Autodesk Inventor part; units mm, degrees
ref_plane "YZ Plane" through (0, 0, 0) normal (1, 0, 0) x (0, 1, 0)
ref_plane "XZ Plane" through (0, 0, 0) normal (0, 1, 0) x (-1, 0, 0)
ref_plane "XY Plane" through (0, 0, 0) normal (0, 0, 1) x (1, 0, 0)
sketch "Sketch1" plane through (0, 0, 0) normal (0, 1, 0) x (-1, 0, 0)
  point P0 (0, 0)
sketch "Sketch2" plane through (0, 0, 0) normal (0, 1, 0) x (-1, 0, 0)
  line L0 (-140.5, 177) -> (140.5, 177)
  line L1 (140.5, 177) -> (140.5, -177)
  line L2 (140.5, -177) -> (-140.5, -177)
  line L3 (-140.5, -177) -> (-140.5, 177)
  line L4 (-140.5, 177) -> (140.5, -177) construction
  line L5 (140.5, 177) -> (-140.5, -177) construction
  point P0 (0, 0)
  dimension "d0" = 354
  dimension "d1" = 281
extrude "Extrusion1" add sketch "Sketch2" along normal blind 11.4
sketch "Sketch3" plane through (0, 0, 0) normal (0, -1, 0) x (1, 0, 0)
  line L0 (-124, -160.5) -> (125.8, -160.5)
  line L1 (125.8, -160.5) -> (125.8, 160.5)
  line L2 (125.8, 160.5) -> (-124, 160.5)
  line L3 (-124, 160.5) -> (-124, -160.5)
  line L4 (-123, -158.8) -> (123, 158.8) construction
  line L5 (123, -158.8) -> (-123, 158.8) construction
  circle A0 centre (-115.5, -152) radius 2
  circle A1 centre (117.3, -152) radius 2
  circle A2 centre (117.3, 152) radius 2
  circle A3 centre (-115.5, 152) radius 2
  line L6 (-140.5, -177) -> (-140.5, 177)
  line L7 (-140.5, 177) -> (140.5, 177)
  line L8 (140.5, -177) -> (-140.5, -177)
  line L9 (140.5, 177) -> (140.5, -177)
  circle A4 centre (-115.5, 0) radius 2
  circle A5 centre (117.3, 0) radius 2
  circle A6 centre (0, 152) radius 2
  circle A7 centre (0, -152) radius 2
  point P0 (0, 0)
  dimension "d189" = 4
  dimension "d190" = 8.5
  dimension "d191" = 8.5
  dimension "d192" = 8.5
  dimension "d193" = 8.5
  dimension "d194" = 8.5
  dimension "d195" = 8.5
  dimension "d196" = 8.5
  dimension "d197" = 8.5
  dimension "d207" = 16.5
  dimension "d208" = 16.5
  dimension "d209" = 16.5
  dimension "d210" = 14.7
  dimension "d211" = 8.5
  dimension "d212" = 354
  dimension "d213" = 177
  dimension "d214" = 8.5
  dimension "d215" = 177
  dimension "d216" = 8.5
  dimension "d217" = 281
  dimension "d218" = 140.5
  dimension "d220" = 140.5
  dimension "d221" = 8.5
extrude "Extrusion2" add sketch "Sketch3" along normal blind 12 contours L3 L2 L1 L0
sketch "Sketch7" plane through (0, -12, 0) normal (0, -1, 0) x (1, 0, 0)
  line L0 (-52.5, 141) -> (105.5, 141)
  line L1 (105.5, 141) -> (105.5, -141)
  line L2 (105.5, -141) -> (-52.5, -141)
  line L3 (-52.5, -141) -> (-52.5, 141)
  line L4 (-52.5, 141) -> (105.5, -141) construction
  line L5 (105.5, 141) -> (-52.5, -141) construction
  line L6 (125.8, -160.5) -> (125.8, 160.5)
  line L7 (-124, -160.5) -> (125.8, -160.5)
  line L8 (-140.5, 177) -> (140.5, 177)
  line L9 (140.5, -177) -> (-140.5, -177)
  line L10 (140.5, 177) -> (140.5, -177)
  point P0 (0, 0)
  dimension "d62" = 158
  dimension "d204" = 36
  dimension "d205" = 36
  dimension "d206" = 35
extrude "Extrusion3" add sketch "Sketch7" along normal blind 31.2
sketch "Sketch8" plane through (0, -43.2, 0) normal (0, -1, 0) x (1, 0, 0)
  line L0 (99.2, 131) -> (81.2, 131)
  line L1 (81.2, 131) -> (81.2, 15)
  line L2 (81.2, 15) -> (99.2, 15)
  line L3 (99.2, 15) -> (99.2, 131)
  line L4 (99.2, 131) -> (81.2, 15) construction
  line L5 (81.2, 131) -> (99.2, 15) construction
  line L6 (105.5, -141) -> (105.5, 141)
  line L7 (105.5, 141) -> (-52.5, 141)
  point P0 (0, 0)
  point P1 (90.2, 73)
  dimension "d67" = 116
  dimension "d68" = 18
  dimension "d69" = 6.3
  dimension "d70" = 10
extrude "Extrusion4" add sketch "Sketch8" along normal blind 1
sketch "Sketch9" plane through (0, -43.2, 0) normal (0, -1, 0) x (1, 0, 0)
  line L0 (100, -71.4) -> (42.15, -71.4)
  line L1 (42.15, -71.4) -> (42.15, -129.25)
  line L2 (42.15, -129.25) -> (100, -129.25)
  line L3 (100, -129.25) -> (100, -71.4)
  line L4 (100, -71.4) -> (42.15, -129.25) construction
  line L5 (42.15, -71.4) -> (100, -129.25) construction
  line L6 (105.5, -141) -> (105.5, 141)
  line L7 (-52.5, -141) -> (105.5, -141)
  point P0 (0, 0)
  point P1 (71.075, -100.325)
  dimension "d73" = 5.5
  dimension "d74" = 57.85
  dimension "d75" = 11.75
  dimension "d76" = 57.85
extrude "Extrusion5" add sketch "Sketch9" along normal blind 1
sketch "Sketch10" plane through (0, -43.2, 0) normal (0, -1, 0) x (1, 0, 0)
  line L0 (105.5, 141) -> (-52.5, 141)
  line L1 (-52.5, 141) -> (-52.5, -141)
  line L2 (-52.5, -141) -> (105.5, -141)
  point P0 (0, 0)
  point P1 (-45.5, 120.2)
  point P2 (-45.5, -119.9)
  dimension "d86" = 20.8
  dimension "d87" = 7
  dimension "d90" = 240.1
  dimension "d95" = 21.1
hole "Hole4" at (-45.5, -43.2, 120.2) at (-45.5, -43.2, -119.9) direction (0, 1, 0) diameter 7 depth 8 tip angle 118
sketch "Sketch11" plane through (0, -43.2, 0) normal (0, -1, 0) x (1, 0, 0)
  line L0 (105.5, 141) -> (-52.5, 141)
  line L1 (-52.5, 141) -> (-52.5, -141)
  line L2 (125.8, 160.5) -> (-124, 160.5)
  point P0 (0, 0)
  point P1 (-45.5, 0)
  dimension "d103" = 141
  dimension "d104" = 7
  dimension "d185" = 160.5
hole "Hole5" at (-45.5, -43.2, 0) direction (0, 1, 0) diameter 7 depth 8 tip angle 118
sketch "Sketch12" plane through (0, -43.2, 0) normal (0, -1, 0) x (1, 0, 0)
  line L0 (105.5, 141) -> (-52.5, 141)
  line L1 (-52.5, 141) -> (-52.5, -141)
  point P0 (0, 0)
  point P1 (-18.7, 37.65)
  point P2 (-18.7, -36.85)
  point P3 (55.8, 37.65)
  point P4 (55.8, -36.85)
  dimension "d112" = 103.35
  dimension "d113" = 33.8
  dimension "d116" = 74.5
  dimension "d119" = 74.5
hole "Hole6" at (-18.7, -43.2, 37.65) at (55.8, -43.2, 37.65) at (55.8, -43.2, -36.85) at (-18.7, -43.2, -36.85) direction (0, 1, 0) diameter 7 depth 8 tip angle 118
sketch "Sketch13" plane through (-52.5, -12, -141) normal (-1, 0, 0) x (0, 0, 1)
  line L0 (223, -24.2) -> (195.5, -24.2)
  line L1 (195.5, -24.2) -> (195.5, -2.2)
  line L2 (195.5, -2.2) -> (223, -2.2)
  line L3 (223, -2.2) -> (223, -24.2)
  line L4 (223, -24.2) -> (195.5, -2.2) construction
  line L5 (195.5, -24.2) -> (223, -2.2) construction
  line L6 (282, 0) -> (282, -31.2)
  line L7 (282, -31.2) -> (0, -31.2)
  point P0 (141, 12)
  point P1 (209.25, -13.2)
  dimension "d122" = 59
  dimension "d123" = 27.5
  dimension "d124" = 22
  dimension "d133" = 7
extrude "Extrusion6" cut sketch "Sketch13" against normal blind 10
sketch "Sketch14" plane through (-52.5, -12, -141) normal (-1, 0, 0) x (0, 0, 1)
  line L0 (142, -11.8) -> (125, -11.8)
  line L1 (125, -11.8) -> (125, -5.6)
  line L2 (125, -5.6) -> (142, -5.6)
  line L3 (142, -5.6) -> (142, -11.8)
  line L4 (142, -11.8) -> (125, -5.6) construction
  line L5 (125, -11.8) -> (142, -5.6) construction
  line L6 (195.5, -24.2) -> (195.5, -2.2)
  line L7 (282, -31.2) -> (0, -31.2)
  line L8 (223, -24.2) -> (195.5, -24.2)
  line L9 (301.5, 0) -> (-19.5, 0)
  line L10 (195.5, -2.2) -> (223, -2.2)
  line L11 (282, 0) -> (282, -31.2)
  point P0 (141, 12)
  point P1 (133.5, -8.7)
  dimension "d128" = 6.2
  dimension "d129" = 17
  dimension "d130" = 19.4
  dimension "d222" = 140
extrude "Extrusion7" cut sketch "Sketch14" against normal blind 1.5
sketch "Sketch15" plane through (-52.5, -12, -141) normal (-1, 0, 0) x (0, 0, 1)
  line L0 (118, -11.8) -> (103, -11.8)
  line L1 (103, -11.8) -> (103, -5.6)
  line L2 (103, -5.6) -> (118, -5.6)
  line L3 (118, -5.6) -> (118, -11.8)
  line L4 (118, -11.8) -> (103, -5.6) construction
  line L5 (103, -11.8) -> (118, -5.6) construction
  line L6 (125, -11.8) -> (125, -5.6)
  line L7 (282, -31.2) -> (0, -31.2)
  point P0 (141, 12)
  point P1 (110.5, -8.7)
  dimension "d136" = 7
  dimension "d137" = 6.2
  dimension "d138" = 15
  dimension "d141" = 19.4
extrude "Extrusion8" cut sketch "Sketch15" against normal blind 1.5
sketch "Sketch16" plane through (-52.5, -12, -141) normal (-1, 0, 0) x (0, 0, 1)
  circle A0 centre (92.5, -12.2) radius 2.5
  line L0 (103, -11.8) -> (103, -5.6)
  line L1 (282, -31.2) -> (0, -31.2)
  circle A1 centre (68, -12.2) radius 2.5
  line L2 (88.375, -16.2) -> (72.125, -16.2)
  line L3 (72.125, -16.2) -> (72.125, -8.2)
  line L4 (72.125, -8.2) -> (88.375, -8.2)
  line L5 (88.375, -8.2) -> (88.375, -16.2)
  line L6 (88.375, -16.2) -> (72.125, -8.2) construction
  line L7 (72.125, -16.2) -> (88.375, -8.2) construction
  point P0 (141, 12)
  point P1 (80.25, -12.2)
  dimension "d142" = 10.5
  dimension "d144" = 5
  dimension "d147" = 24.5
  dimension "d223" = 19
  dimension "d224" = 12.25
  dimension "d225" = 19
  dimension "d226" = 16.25
  dimension "d227" = 8
extrude "Extrusion9" add sketch "Sketch16" along normal blind 5
sketch "Sketch20" plane through (0, -12, 0) normal (0, -1, 0) x (1, 0, 0)
  circle A0 centre (-59, 120) radius 2
  circle A1 centre (-59, 0) radius 2
  circle A2 centre (-59, -120) radius 2
  line L0 (-52.5, -141) -> (-52.5, 141)
  circle A3 centre (-115.5, 152) radius 2
  point P0 (0, 0)
  dimension "d228" = 21
  dimension "d229" = 6.5
  dimension "d230" = 6.5
  dimension "d231" = 6.5
  dimension "d232" = 21
  dimension "d233" = 240
  dimension "d234" = 120
extrude "Extrusion11" cut sketch "Sketch20" against normal blind 10 contours A0 | A1 | A2
equation "\"d191\" = d190"
equation "\"d192\" = d190"
equation "\"d193\" = d190"
equation "\"d194\" = d190"
equation "\"d195\" = d190"
equation "\"d196\" = d190"
equation "\"d197\" = d190"
equation "\"d209\" = d208"
equation "\"d211\" = d190"
equation "\"d213\" = 0.5 * d212"
equation "\"d214\" = d190"
equation "\"d215\" = d213"
equation "\"d216\" = d190"
equation "\"d218\" = 0.5 * d217"
equation "\"d220\" = d218"
equation "\"d221\" = d190"
equation "\"d205\" = d204"
equation "\"d230\" = d229"
equation "\"d231\" = d229"
equation "\"d232\" = d228"
equation "\"d234\" = 0.5 * d233"
properties part number "LCDScreen"
The listing builds one solid part. Answer for the finished solid, in the listing's coordinates (mm). A direction names the side the tool comes from. Give positions to 0.01 mm unless a question says otherwise; leave off trailing zeros. Loops run counter-clockwise (first coordinate to the right, second up) from the corner with the lowest first, then second, coordinate; pieces in that order, holes last. Notation, with made-up numbers: M 89,-0.5 L 104,-0.5 A32 ccw 104,25.5 Z; hole C -18,-19.5 d10. An arc over 180 degrees is marked long. One line per item, written item: value.
Q1. Find the intervals of material crossed by line 1 (X direction, y = -8.5, z = 152); line 2 (Z direction, x = -59, y = -5.75); line 3 (Z direction, x = 117.3, y = -3.5), in increasing order. Write a range as from..to.
Working result:
line 1: x = -124..-117.5, -113.5..-2, 2..115.3, 119.3..125.8
line 2: z = -160.5..-122, -118..-2, 2..118, 122..160.5
line 3: z = -160.5..-154, -150..-2, 2..150, 154..160.5
Q2. A cutting plane is placed at D-D on z = 25. Determine the outline of the cut face in (x, y).
Working result:
outline: M -140.5,0 L -124,0 L -124,-12 L -52.5,-12 L -52.5,-43.2 L 81.2,-43.2 L 81.2,-44.2 L 99.2,-44.2 L 99.2,-43.2 L 105.5,-43.2 L 105.5,-12 L 125.8,-12 L 125.8,0 L 140.5,0 L 140.5,11.4 L -140.5,11.4 Z
Q3. Determine the mould class of faces 1 (the face through (-45.73, -33.46, -120.46)), 2 (the face through (56.4, -33.46, 37.73)), 3 (the face through (2, 6, 177)), 4 (the face through (-124.2, 0, -12.3)) for opening direction Z: +Z half, -Z half, draft (parallel to the pull), parting line (faces both ways), or undercut.
Working result:
face 1: undercut
face 2: undercut
face 3: +Z half
face 4: draft
Q4. A cutting plane is placed at C-C on z = 135. Determine the outline of the cut face in (x, y), then the cut area to 3 significant figures.
Working result:
outline: M -140.5,0 L -124,0 L -124,-12 L -52.5,-12 L -52.5,-43.2 L 105.5,-43.2 L 105.5,-12 L 125.8,-12 L 125.8,0 L 140.5,0 L 140.5,11.4 L -140.5,11.4 Z
area: 11,100 mm^2
Q5. For faces 5 (the face through (90, -44.2, 74)), 6 (the face through (25, -27, 141)), 7 (the face through (-140.5, 6, 2)), 8 (the face through (-15.595, -39.144, -38.465)), 9 (the face through (-48, -36.2, 68)), determine the directions among +Z, -Z, +X, -X, +Y, -Y from which every point of the face is accessible in a straight line to the end or side of a thin tool.
Working result:
face 5: +Z, -Z, +X, -X, -Y
face 6: +Z, +X, -X, -Y
face 7: +Z, -Z, -X, +Y, -Y
face 8: -Y
face 9: -X
Q6. Flat-ended cylindrical pins translate along their axes: P1, Ø4, axis at y = -23.5, z = -49, coming from the -X side; P2, Ø1.1, axis at x = 86.5, y = -44, coming from the +Z side; P3, Ø0.5, axis at y = -43.5, z = 67.5, coming from the +X side. Find the tip coordinate at first contact, or state that the pin passes through.
Working result:
P1: stops at x = -57.5
P2: stops at z = 131
P3: stops at x = 99.2
Q7. A cutting plane is placed at B-B on x = -10.5. Determine the outline of the cut face in (y, z).
Working result:
outline: M -43.2,-141 L -12,-141 L -12,-160.5 L 0,-160.5 L 0,-177 L 11.4,-177 L 11.4,177 L 0,177 L 0,160.5 L -12,160.5 L -12,141 L -43.2,141 Z
Q8. A cutting plane is placed at A-A on z = -105. Determine the outline of the cut face in (x, y).
Working result:
outline: M -140.5,0 L -124,0 L -124,-12 L -52.5,-12 L -52.5,-43.2 L 42.15,-43.2 L 42.15,-44.2 L 100,-44.2 L 100,-43.2 L 105.5,-43.2 L 105.5,-12 L 125.8,-12 L 125.8,0 L 140.5,0 L 140.5,11.4 L -140.5,11.4 Z
